The drawing under review shows one solid part. Ordinate dimensions are in mm from its lowest x, y, z. A direction names the side the tool comes from. Coordinates: 2 decimals unless noted, no trailing zeros. Loops run counter-clockwise (first coordinate to the right, second up) from the corner with the lowest first, then second, coordinate; pieces in that order, holes last. Notation, with made-up numbers: (10, 77) - (39, 77) arc R18 cw to (39, 108) - close; hole circle Ø11 at (7.25, 45.25). An arc over 180 degrees is marked (long way). Use one line per item in the form item = value. Start each with the question number.
1. Draft analysis for pull direction X (two halves, no side actions). For the marked faces 1, 2, 3 and 4, state which applies: +X half, -X half, draft (parallel to the pull), parting line (faces both ways), or undercut.
2. Add section C-C on x = 16.75. Give the boundary of the cut face in (y, z).
3. Machinability: for the marked faces 5 and 6, which of the approach directions +Z, -Z, +X, -X, +Y, -Y give a long, thin tool a straight path to every point of the face, cutting with its end or side? Answer none if there is none.
4. For pin 1 Ø6 at (x, y) = (14, 16.5) entering from +Z (1 decimal), flat-tipped, find the tip position at first contact; note if it passes through.
5. To check wall thickness, follow probe 1 along X at (y, z) = (22.9, 2.5); probe 2 along Z at (x, y) = (8, 21.4); probe 3 along Y at (x, z) = (12.5, 0.7). State the ranges of each line that lie inside material, in increasing order.
6. Add section A-A on x = 12.5. Give the boundary of the cut face in (y, z), and give its area (3 significant figures).
7. Add section D-D on x = 8. Give the boundary of the cut face in (y, z).
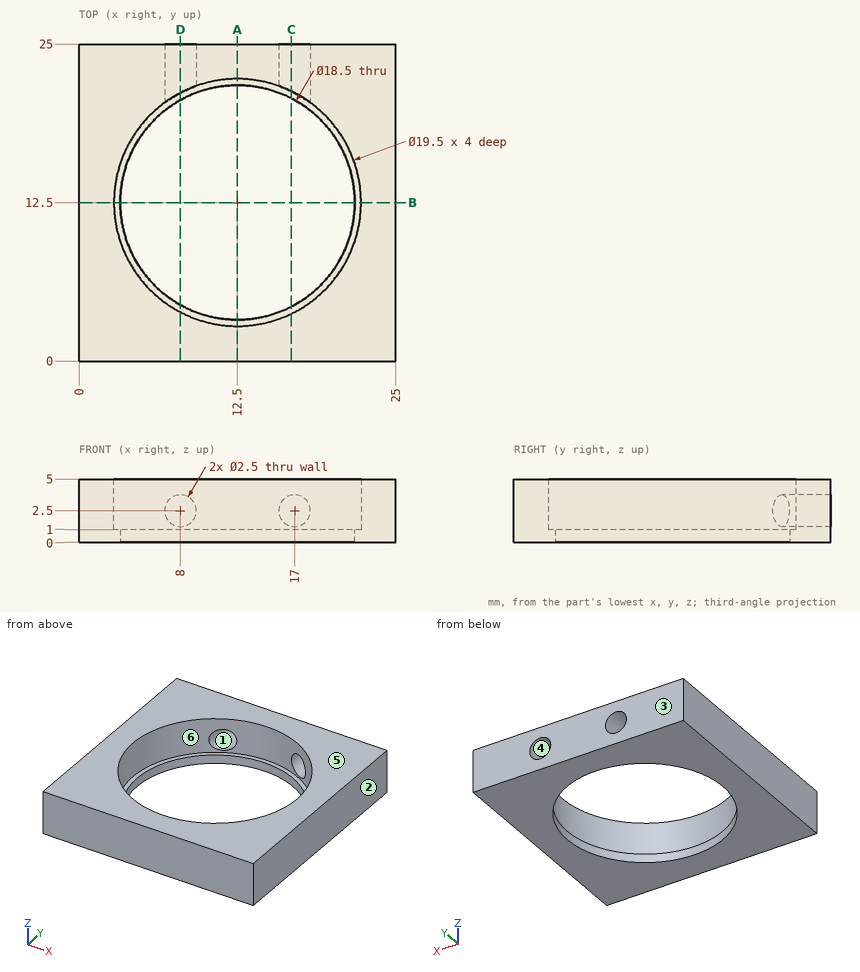
Conclusion:
q1.face_1 = undercut
q1.face_2 = +X half
q1.face_3 = draft
q1.face_4 = undercut
q2.outline = (0, 0) - (4.28, 0) - (4.28, 1) - (3.73, 1) - (3.73, 5) - (0, 5) - close; (20.72, 0) - (25, 0) - (25, 1.28) - (21.27, 1.28) - (21.27, 1) - (20.72, 1) - close; (21.27, 3.72) - (25, 3.72) - (25, 5) - (21.27, 5) - close
q3.face_5 = +Z, +X, -X, +Y, -Y
q3.face_6 = +Z
q4.pin_1 = through
q5.probe_1 = 0 to 6.75, 9.25 to 15.75, 18.25 to 25
q5.probe_2 = 0 to 1.25, 3.75 to 5
q5.probe_3 = 0 to 3.25, 21.75 to 25
q6.outline = (0, 0) - (3.25, 0) - (3.25, 1) - (2.75, 1) - (2.75, 5) - (0, 5) - close; (21.75, 0) - (25, 0) - (25, 5) - (22.25, 5) - (22.25, 1) - (21.75, 1) - close
q6.area = 28.5 mm^2
q7.outline = (0, 0) - (4.42, 0) - (4.42, 1) - (3.85, 1) - (3.85, 5) - (0, 5) - close; (20.58, 0) - (25, 0) - (25, 1.25) - (21.15, 1.25) - (21.15, 1) - (20.58, 1) - close; (21.15, 3.75) - (25, 3.75) - (25, 5) - (21.15, 5) - close
